Model file for the job. Use its own axes, mm. A direction names the side the tool comes from. Give positions to 0.01 mm unless a question says otherwise; leave off trailing zeros. Loops run counter-clockwise (first coordinate to the right, second up) from the corner with the lowest first, then second, coordinate; pieces in that order, holes last. Notation, with made-up numbers: M 57,77.5 L 109,77.5 A33 cw 109,115.5 Z; hole C 15.25,59.25 d6. An arc over 180 degrees is marked long. Answer in a Markdown table with one row per item.
Autodesk Inventor part; units mm, degrees
ref_plane "YZ Plane" through (0, 0, 0) normal (1, 0, 0) x (0, 1, 0)
ref_plane "XZ Plane" through (0, 0, 0) normal (0, 1, 0) x (-1, 0, 0)
ref_plane "XY Plane" through (0, 0, 0) normal (0, 0, 1) x (1, 0, 0)
sketch "Эскиз1" plane through (0, 0, 0) normal (0, 0, 1) x (1, 0, 0)
  line L0 (-26.0621, -17.2379) -> (-22.2379, -21.0621)
  arc A0 (-22.2379, -21.0621) -> (-22.0257, -21.15) centre (-22.0257, -20.85) ccw
  line L1 (-22.0257, -21.15) -> (12.0257, -21.15)
  arc A1 (12.0257, -21.15) -> (12.2379, -21.0621) centre (12.0257, -20.85) ccw
  line L2 (12.2379, -21.0621) -> (16.0621, -17.2379)
  arc A2 (16.0621, -17.2379) -> (16.15, -17.0257) centre (15.85, -17.0257) ccw
  line L3 (16.15, -17.0257) -> (16.15, 17.0257)
  arc A3 (16.15, 17.0257) -> (16.0621, 17.2379) centre (15.85, 17.0257) ccw
  line L4 (16.0621, 17.2379) -> (12.2379, 21.0621)
  arc A4 (12.2379, 21.0621) -> (12.0257, 21.15) centre (12.0257, 20.85) ccw
  line L5 (12.0257, 21.15) -> (-22.0257, 21.15)
  arc A5 (-22.0257, 21.15) -> (-22.2379, 21.0621) centre (-22.0257, 20.85) ccw
  line L6 (-22.2379, 21.0621) -> (-26.0621, 17.2379)
  arc A6 (-26.0621, 17.2379) -> (-26.15, 17.0257) centre (-25.85, 17.0257) ccw
  line L7 (-26.15, 17.0257) -> (-26.15, -17.0257)
  arc A7 (-26.15, -17.0257) -> (-26.0621, -17.2379) centre (-25.85, -17.0257) ccw
  circle A8 centre (-5, 0) radius 11
  circle A9 centre (-20.5, 15.5) radius 1.25
  circle A10 centre (10.5, 15.5) radius 1.25
  circle A11 centre (10.5, -15.5) radius 1.25
  circle A12 centre (-20.5, -15.5) radius 1.25
  circle A13 centre (20.65, -19.15) radius 1.75
  circle A14 centre (20.65, 0.85) radius 1.75
  circle A15 centre (20.65, 20.85) radius 1.75
  circle A16 centre (20.65, 40.85) radius 1.75
  line L8 (-246.5621, -17.2379) -> (-242.7379, -21.0621)
  arc A17 (-242.7379, -21.0621) -> (-242.5257, -21.15) centre (-242.5257, -20.85) ccw
  line L9 (-242.5257, -21.15) -> (-208.4743, -21.15)
  arc A18 (-208.4743, -21.15) -> (-208.2621, -21.0621) centre (-208.4743, -20.85) ccw
  line L10 (-208.2621, -21.0621) -> (-204.4379, -17.2379)
  arc A19 (-204.4379, -17.2379) -> (-204.35, -17.0257) centre (-204.65, -17.0257) ccw
  line L11 (-204.35, -17.0257) -> (-204.35, 17.0257)
  arc A20 (-204.35, 17.0257) -> (-204.4379, 17.2379) centre (-204.65, 17.0257) ccw
  line L12 (-204.4379, 17.2379) -> (-208.2621, 21.0621)
  arc A21 (-208.2621, 21.0621) -> (-208.4743, 21.15) centre (-208.4743, 20.85) ccw
  line L13 (-208.4743, 21.15) -> (-242.5257, 21.15)
  arc A22 (-242.5257, 21.15) -> (-242.7379, 21.0621) centre (-242.5257, 20.85) ccw
  line L14 (-242.7379, 21.0621) -> (-246.5621, 17.2379)
  arc A23 (-246.5621, 17.2379) -> (-246.65, 17.0257) centre (-246.35, 17.0257) ccw
  line L15 (-246.65, 17.0257) -> (-246.65, -17.0257)
  arc A24 (-246.65, -17.0257) -> (-246.5621, -17.2379) centre (-246.35, -17.0257) ccw
  circle A25 centre (-225.5, 0) radius 11
  circle A26 centre (-241, 15.5) radius 1.25
  circle A27 centre (-210, 15.5) radius 1.25
  circle A28 centre (-210, -15.5) radius 1.25
  circle A29 centre (-241, -15.5) radius 1.25
  circle A30 centre (-251.15, -19.15) radius 1.75
  circle A31 centre (-251.15, 0.85) radius 1.75
  circle A32 centre (-251.15, 20.85) radius 1.75
  circle A33 centre (-251.15, 40.85) radius 1.75
  line L16 (-255.45, -29.15) -> (-246.85, -29.15)
  line L17 (-255.65, -29.15) -> (-255.65, 270.85)
  line L18 (25.15, 270.85) -> (25.15, -29.15)
  line L19 (25.15, -29.15) -> (-255.65, -29.15)
  line L20 (-255.65, -29.15) -> (-255.65, 45.35)
  line L21 (-255.65, 45.35) -> (25.15, 45.35)
  line L22 (25.15, 45.35) -> (25.15, -29.15)
  point P0 (25.15, 45.35)
  dimension "d15" = 4.5
extrude "Выдавливание1" add sketch "Эскиз1" along normal blind 6 contours A7 L7 A6 L6 A5 L5 A4 L4 A3 L3 A2 L2 A1 L1 A0 L0 | A24 L15 A23 L14 A22 L13 A21 L12 A20 L11 A19 L10 A18 L9 A17 L8 | L19 L17 L21 L18 L16
sketch "Эскиз2" plane through (0, 0, 6) normal (0, 0, 1) x (1, 0, 0)
  circle A0 centre (20.65, 40.85) radius 1.75
  circle A1 centre (5.65, 40.85) radius 2.6
  circle A2 centre (-236.15, 40.85) radius 2.6
  circle A3 centre (-251.15, 40.85) radius 1.75
  point P0 (0, 0)
  dimension "d16" = 5.2
  dimension "d17" = 15
  dimension "d18" = 5.2
  dimension "d19" = 15
extrude "Выдавливание2" cut sketch "Эскиз2" against normal blind 6
sketch "Эскиз3" plane through (0, 0, 0) normal (0, 0, -1) x (-1, 0, 0)
  circle A0 centre (115.25, -18.05) radius 2.55
  circle A1 centre (115.25, 1.95) radius 2.55
  line L0 (255.65, 45.35) -> (255.65, -29.15)
  point P0 (0, 0)
  dimension "d25" = 5.1
  dimension "d26" = 140.4
  dimension "d27" = 140.4
extrude "Выдавливание3" cut sketch "Эскиз3" against normal blind 10
sketch "Эскиз4" plane through (0, 0, 6) normal (0, 0, 1) x (1, 0, 0)
  circle A0 centre (-177.15, -2.65) radius 5 construction
  line L0 (-177.15, -2.65) -> (-177.15, -29.15) construction
  line L1 (-255.65, -29.15) -> (25.15, -29.15) construction
  circle A1 centre (-177.15, -9.15) radius 5
  point P0 (0, 0)
  dimension "d30" = 10
  dimension "d31" = 20
extrude "Выдавливание4" cut sketch "Эскиз4" against normal blind 10
sketch "Эскиз5" plane through (0, 0, 6) normal (0, 0, 1) x (1, 0, 0)
  circle A0 centre (-20.5, 15.5) radius 1.25 construction
  circle A1 centre (-20.5, -15.5) radius 1.25 construction
  circle A2 centre (-20.5, -15.5) radius 1.25
  circle A3 centre (-20.5, 15.5) radius 1.25
  line L0 (-20.5, -15.5) -> (-20.5, 15.5) construction
  line L1 (-60.8, -17.65) -> (-35.5, -17.65)
  line L2 (-35.5, -17.65) -> (-35.5, -0.65)
  line L3 (-35.5, -0.65) -> (-60.8, -0.65)
  line L4 (-60.8, -0.65) -> (-60.8, -17.65)
  line L5 (-60.8, -17.65) -> (-35.5, -0.65) construction
  line L6 (-35.5, -17.65) -> (-60.8, -0.65) construction
  circle A4 centre (-58.8, -20.9) radius 1.35
  line L7 (-48.15, -9.15) -> (-48.15, -2.4897)
  line L8 (-48.15, -9.15) -> (-50.139, -9.15)
  circle A5 centre (-37.5, -20.9) radius 1.35
  circle A6 centre (-58.8, 2.6) radius 1.35
  circle A7 centre (-37.5, 2.6) radius 1.35
  line L9 (-255.65, -29.15) -> (25.15, -29.15)
  point P0 (0, 0)
  dimension "d33" = 17
  dimension "d39" = 2.7
  dimension "d40" = 3.25
  dimension "d41" = 2
  dimension "d45" = 25.3
  dimension "d46" = 20
extrude "Выдавливание5" cut sketch "Эскиз5" against normal blind 10
sketch "Эскиз6" plane through (0, 0, 6) normal (0, 0, 1) x (1, 0, 0)
  line L0 (-60.8, -17.65) -> (-60.8, -0.65) construction
  line L1 (-60.8, -9.15) -> (-101.8454, -9.15) construction
  circle A0 centre (-75.8, -19.15) radius 2.55
  circle A1 centre (-75.8, 0.85) radius 2.55
  line L2 (-75.8, 0.85) -> (-75.8, -20.3687) construction
  line L3 (-101.8454, -9.15) -> (-167.9603, -9.15) construction
  circle A2 centre (-140.8, -9.15) radius 11
  point P0 (0, 0)
  dimension "d47" = 5.1
  dimension "d48" = 5.1
  dimension "d49" = 10
  dimension "d50" = 10
  dimension "d51" = 15
  dimension "d54" = 22
  dimension "d55" = 65
extrude "Выдавливание6" cut sketch "Эскиз6" against normal blind 10
properties part number "креп_мотора" material "Древесина (береза)"
(1) Which spindle directions (+Z, -Z, +X, -X, +Y, -Y) get a long thin tool onto all of the face, cutting with end or side? Do faces 1 (the flat face through (-117, 45.35, 3)), 2 (the flat face through (-48, -17.65, 3)). Say none if no direction does.
Established:
| item | result |
|---|---|
| face 1 | +Z, -Z, +X, -X, +Y |
| face 2 | +Z, -Z |
(2) Saw through at D-D, the plane z = 4.15. Count the separate pieces of the cut face and the enclosed holes in it, and give its area (3 significant figures).
Established:
| item | result |
|---|---|
| separate pieces | 1 |
| enclosed holes | 31 |
| area | 19,000 mm2 |
(3) Flat gauge pin, fed straight in: P1, Ø3, axis at x = 5.65, y = 40.85, coming from the -Z side. Where does the tip first touch, or does it go through?
Established:
| item | result |
|---|---|
| P1 | passes through |
(4) Saw through at A-A, the plane x = -5. Give the cut face in (y, z), and give its area (3 significant figures).
Established:
| item | result |
|---|---|
| outline | M -29.15,0 L -11,0 L -11,6 L -29.15,6 Z; M 11,0 L 45.35,0 L 45.35,6 L 11,6 Z |
| area | 315 mm2 |
(5) Saw through at B-B, the plane y = 8.5. Give the cut face in (x, z), and give its area (3 significant figures).
Established:
| item | result |
|---|---|
| outline | M -255.65,0 L -232.48,0 L -232.48,6 L -255.65,6 Z; M -218.52,0 L -11.98,0 L -11.98,6 L -218.52,6 Z; M 1.98,0 L 25.15,0 L 25.15,6 L 1.98,6 Z |
| area | 1,520 mm2 |
(6) Saw through at C-C, the plane x = -177.15. Give the cut face in (y, z).
Established:
| item | result |
|---|---|
| outline | M -29.15,0 L -14.15,0 L -14.15,6 L -29.15,6 Z; M -4.15,0 L 45.35,0 L 45.35,6 L -4.15,6 Z |
(7) Mould opens along X. For faces 3 (the flat face through (-113, -29.15, 3)), 4 (the cylindrical face through (-117.68, -17.28, 2.96)), 5 (the cylindrical face through (5.161, 4.213, 2.958)), 6 (the flat face through (-255.65, 8, 3)) say: pulls with the +X half, pulls with the -X half, needs draft (parallel to the pull), parting line crosses it, or undercut.
Established:
| item | result |
|---|---|
| face 3 | needs draft |
| face 4 | undercut |
| face 5 | undercut |
| face 6 | pulls with the -X half |
(8) Wall check: L1, parallel to Y at x = -241, z = 3.5; L2, parallel to Y at x = -251.15, z = 3.3; L3, parallel to Y at x = -225.5, z = 1.35. Give the ranges that are in metal, low to high.
Established:
| item | result |
|---|---|
| L1 | y = -29.15 to -16.75, -14.25 to 14.25, 16.75 to 45.35 |
| L2 | y = -29.15 to -20.9, -17.4 to -0.9, 2.6 to 19.1, 22.6 to 39.1, 42.6 to 45.35 |
| L3 | y = -29.15 to -11, 11 to 45.35 |
